The figure shows three views and two pictorial views of one solid part (mm, origin at its lowest corner). Answer the questions. Coordinates: 2 decimals unless noted, no trailing zeros. Loops run counter-clockwise (first coordinate to the right, second up) from the corner with the lowest first, then second, coordinate; pieces in that order, holes last.
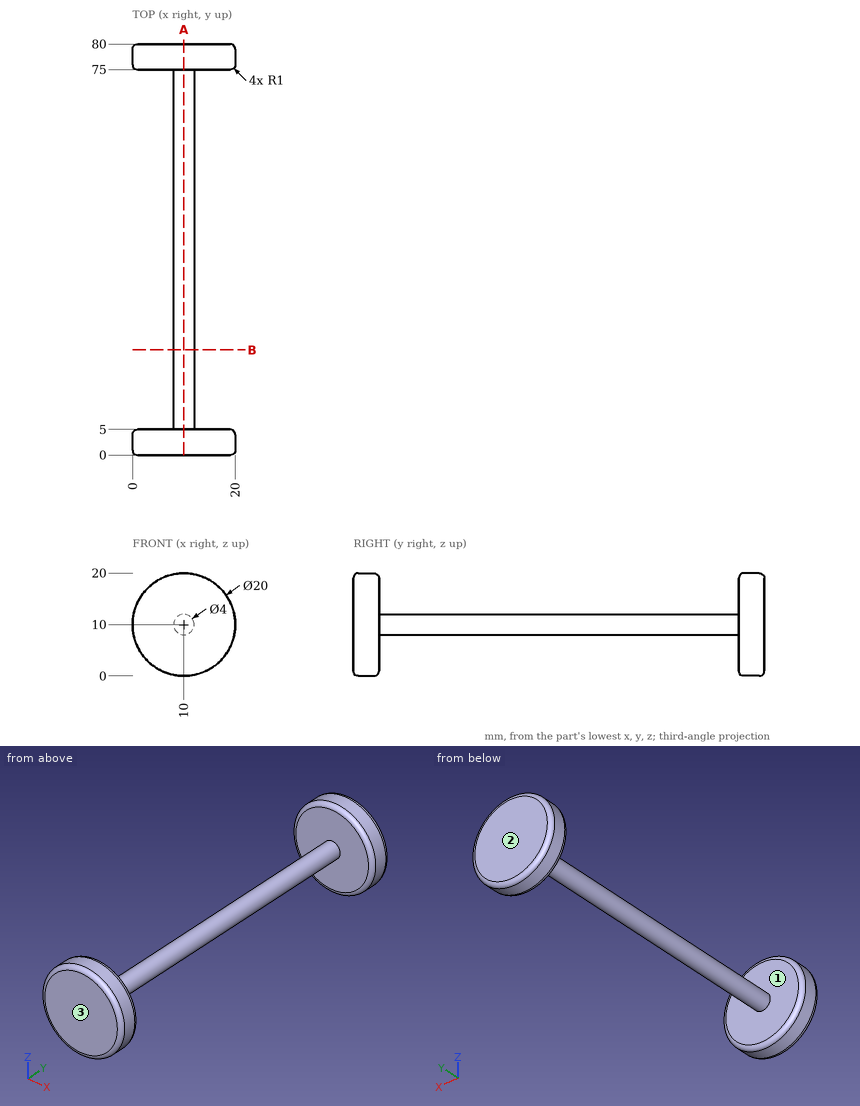
1. A cutting plane is placed at B-B, the plane y = 20.5. Give the vertices of the cut face in (x, z), then the cut area to 3 significant figures.
2. Straight lines are drawn through the part: probe 1 along Y at (x, z) = (3.75, 5.5); probe 2 along Z at (x, y) = (9.75, 59). For each, find the intervals that lie inside material, in ascending order.
3. A cutting plane is placed at A-A, the plane x = 10. Give the vertices of the cut face in (y, z), then the cut area to 3 significant figures.
4. Determine the mould class of the marked faces 1, 2 and 3 for opening direction Y: released by +Y, released by -Y, zero draft, split by the parting line, or undercut.
5. Each of these flat-tipped pins is pushed along its axis until it touches: P1, Ø5, axis at x = 9, y = 62, coming from the -Z side; P2, Ø5, axis at x = 6, y = 29.5, coming from the -Z side; P3, Ø6, axis at y = 64, z = 6.5, coming from the +X side. Where does it stop, or does it pass through?
Answers below:
1. outline: circle Ø4 at (10, 10)
1. area: 12.6 mm2
2. probe 1: y = 0 to 5, 75 to 80
2. probe 2: z = 8.02 to 11.98
3. outline: (0, 1) arc R1 ccw to (1, 0) - (4, 0) arc R1 ccw to (5, 1) - (5, 8) - (75, 8) - (75, 1) arc R1 ccw to (76, 0) - (79, 0) arc R1 ccw to (80, 1) - (80, 19) arc R1 ccw to (79, 20) - (76, 20) arc R1 ccw to (75, 19) - (75, 12) - (5, 12) - (5, 19) arc R1 ccw to (4, 20) - (1, 20) arc R1 ccw to (0, 19) - close
3. area: 478 mm2
4. face 1: undercut
4. face 2: released by +Y
4. face 3: released by -Y
5. P1: stops at z = 8
5. P2: stops at z = 8.68
5. P3: stops at x = 11.94
